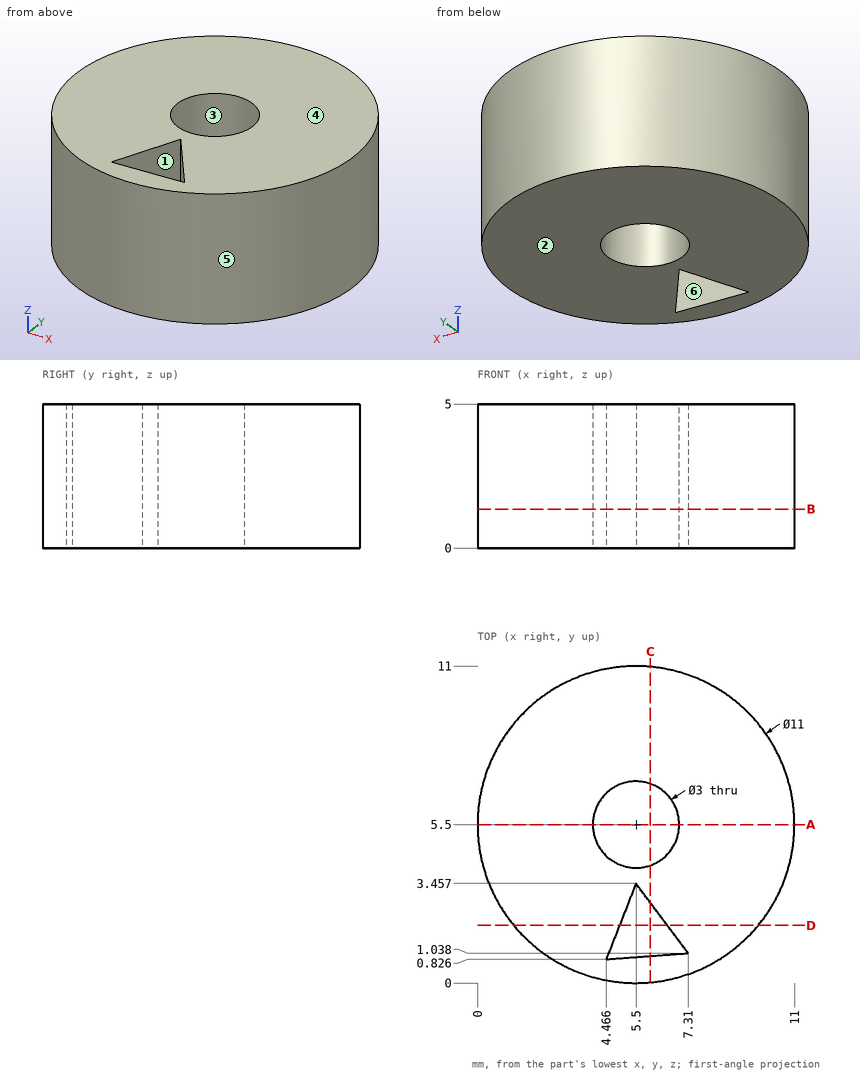
Answer from the drawing. Dimensions are ordinates in mm from the lowest x, y and z of the part. A direction names the side the tool comes from. Give positions to 0.01 mm unless a question says otherwise; leave off trailing zeros. Order: outer loops, then holes, each group sorted by start corner. A loop starts at its lowest first (then second) coordinate and runs counter-clockwise, first axis right, second up.
(1) For the marked faces 1 and 2, determine the directions among +Z, -Z, +X, -X, +Y, -Y from which every point of the face is accessible in a straight line to the end or side of a thin tool.
(2) Find section A-A (y = 5.5). Give the vertices of the cut face in (x, z), plus the area to 3 significant figures.
(3) Find section C-C (x = 6). Give the vertices of the cut face in (y, z) (1 decimal).
(4) For a pull along X with two mould halves and no side action, classify the marked faces 3, 4, 5 and 6 as released by +X, released by -X, zero draft, split by the parting line, or undercut.
(5) Given pin 1 (2.5 mm diameter, centred on x = 5.5, y = 5.5, fed in from +Z); pin 2 (2 mm diameter, centred on x = 2.5, z = 3.5, fed in from +Y), each flat-ended and moving along its own axis, determine where each tip first touches the part or whether it passes through.
(6) Find section B-B (z = 1.35). Give the vertices of the cut face in (x, y).
(7) Straight lines are drawn through the part: L1, parallel to X at y = 2, z = 2.4; L2, parallel to X at y = 4.5, z = 2.05; L3, parallel to Y at x = 10, z = 2.35 (1 decimal). For each, find the intervals that lie inside material, in ascending order.
(8) Find section D-D (y = 2). Give the vertices of the cut face in (x, z).
Result sheet:
1. face 1: +Z, -Z
1. face 2: -Z, +X, -X, +Y, -Y
2. outline: (0, 0) - (4, 0) - (4, 5) - (0, 5) - close; (7, 0) - (11, 0) - (11, 5) - (7, 5) - close
2. area: 40.0 mm2
3. outline: (0, 0) - (0.9, 0) - (0.9, 5) - (0, 5) - close; (2.8, 0) - (4.1, 0) - (4.1, 5) - (2.8, 5) - close; (6.9, 0) - (11, 0) - (11, 5) - (6.9, 5) - close
4. face 3: undercut
4. face 4: zero draft
4. face 5: split by the parting line
4. face 6: undercut
5. pin 1: passes through
5. pin 2: stops at y = 10.62
6. outline: circle Ø11 at (5.5, 5.5); hole circle Ø3 at (5.5, 5.5); hole (4.47, 0.83) - (7.31, 1.04) - (5.5, 3.46) - close
7. L1: x = 1.26 to 4.93, 6.59 to 9.74
7. L2: x = 0.09 to 4.38, 6.62 to 10.91
7. L3: y = 2.3 to 8.7
8. outline: (1.26, 0) - (4.93, 0) - (4.93, 5) - (1.26, 5) - close; (6.59, 0) - (9.74, 0) - (9.74, 5) - (6.59, 5) - close
